The model under review builds one solid part; all positions refer to its coordinate system, in mm. Face numbers are marked on the shaded views. A direction names the side the tool comes from. Coordinates: 2 decimals unless noted, no trailing zeros. Order: outer loops, then holes, each group sorted by start corner. A loop starts at its lowest first (then second) coordinate and runs counter-clockwise, first axis right, second up. Notation, with made-up numbers: M -8,28 L 16,28 A13 ccw 16,52 Z; hole C 28.25,77 d4. An arc over 180 degrees is marked long. One line per item, written item: value.
Autodesk Inventor part; units mm, degrees
ref_plane "YZ Plane" through (0, 0, 0) normal (1, 0, 0) x (0, 1, 0)
ref_plane "XY Plane" through (0, 0, 0) normal (0, 0, 1) x (1, 0, 0)
sketch "Sketch1" plane through (0, 0, 0) normal (0, 0, 1) x (1, 0, 0)
  circle A0 centre (10.05, 11) radius 1.75
  arc A1 (13.575, 6.828427) -> (12.575, 7) centre (12.575, 4) ccw
  line L0 (13.575, 25.055513) -> (13.575, 6.828427)
  arc A2 (13.582607, 25.229787) -> (13.575, 25.055513) centre (15.575, 25.055513) ccw
  arc A3 (12.575, 25.055513) -> (13.582607, 25.229787) centre (12.575, 28.055513) ccw
  line L1 (7.525, 25.055513) -> (12.575, 25.055513)
  arc A4 (6.525, 25.227086) -> (7.525, 25.055513) centre (7.525, 28.055513) ccw
  line L2 (6.525, 6.828427) -> (6.525, 25.227086)
  arc A5 (7.525, 7) -> (6.525, 6.828427) centre (7.525, 4) ccw
  line L3 (12.575, 7) -> (7.525, 7)
  circle A6 centre (10.05, 21.055513) radius 1.75
  line L4 (10.05, 18.055513) -> (22.075, 18.055513)
  line L5 (22.075, 18.055513) -> (22.075, 56.065748)
  circle A7 centre (18.075, 30.055513) radius 1.75
  circle A8 centre (59, 30.055513) radius 1.75
  circle A9 centre (50.975, 2) radius 1.75
  circle A10 centre (10.05, 2) radius 1.75
  line L6 (3.525, -2) -> (3.525, 34.055513)
  arc A11 (3.525, -2) -> (63.525, -2) centre (33.525, 16.027756) ccw
  line L7 (63.525, 34.055513) -> (63.525, -2)
  arc A12 (63.525, 34.055513) -> (3.525, 34.055513) centre (33.525, 16.027756) ccw
  arc A13 (30.525, 56.680798) -> (-6.475, 36.055513) centre (29.281483, 15.411497) ccw
  arc A14 (30.525, 58.681663) -> (-8.207051, 37.055513) centre (29.281483, 15.411497) ccw
  line L8 (16.075, 54.530422) -> (16.075, 24.055513)
  line L9 (16.075, 24.055513) -> (10.05, 24.055513)
  arc A15 (10.05, 24.055513) -> (10.05, 18.055513) centre (10.05, 21.055513) ccw
  line L10 (-6.475, 36.055513) -> (-8.207051, 37.055513)
  line L11 (30.525, 56.680798) -> (30.525, 58.681663)
  line L12 (15.575, 28.055513) -> (15.575, 32.055513)
  point P0 (0, 0)
  point P1 (30.525, 57.681231)
  dimension "d0" = 6
  dimension "d1" = 6
  dimension "d2" = 3
  dimension "d3" = 2
  dimension "d4" = 2
  dimension "d5" = 0.5
  dimension "d6" = 60
  dimension "d22" = 10
  dimension "d23" = 2
sketch "Sketch1 outline for Extrusion1" plane through (0, 0, 0) normal (0, 0, 1) x (1, 0, 0)
  arc A0 (-6.475, 36.055513) -> (16.075, 54.530422) centre (29.281483, 15.411497) cw
  line L0 (16.075, 54.530422) -> (16.075, 24.055513)
  line L1 (16.075, 24.055513) -> (10.05, 24.055513)
  arc A1 (10.05, 24.055513) -> (10.05, 18.055513) centre (10.05, 21.055513) ccw
  line L2 (10.05, 18.055513) -> (22.075, 18.055513)
  line L3 (22.075, 18.055513) -> (22.075, 56.065748)
  arc A2 (22.075, 56.065748) -> (30.525, 56.680798) centre (29.281483, 15.411497) cw
  line L4 (30.525, 56.680798) -> (30.525, 58.681663)
  arc A3 (30.525, 58.681663) -> (-8.207051, 37.055513) centre (29.281483, 15.411497) ccw
  line L5 (-8.207051, 37.055513) -> (-6.475, 36.055513)
  circle A4 centre (10.05, 21.055513) radius 1.75
extrude "Extrusion1" add sketch "Sketch1 outline for Extrusion1" along normal blind 6
sketch "Sketch2" plane through (0, 0, 0) normal (0, 0, -1) x (-1, 0, 0)
  circle A0 centre (-10.05, 21.055513) radius 1.75
  arc A1 (6.475, 36.055513) -> (-16.075, 54.530422) centre (-29.281483, 15.411497) ccw
  line L0 (8.207051, 37.055513) -> (6.475, 36.055513)
  arc A2 (8.207051, 37.055513) -> (-30.525, 58.681663) centre (-29.281483, 15.411497) ccw
  line L1 (-30.525, 56.680798) -> (-30.525, 58.681663)
  arc A3 (-22.075, 56.065748) -> (-30.525, 56.680798) centre (-29.281483, 15.411497) ccw
  line L2 (-22.075, 18.055513) -> (-22.075, 56.065748)
  line L3 (-10.05, 18.055513) -> (-22.075, 18.055513)
  arc A4 (-10.05, 18.055513) -> (-10.05, 24.055513) centre (-10.05, 21.055513) ccw
  line L4 (-16.075, 24.055513) -> (-10.05, 24.055513)
  line L5 (-16.075, 54.530422) -> (-16.075, 24.055513)
  line L6 (-16.075, 54.530422) -> (-16.075, 24.055513)
  line L7 (-10.05, 18.055513) -> (-22.075, 18.055513)
  line L8 (-19.575, 34.055513) -> (-12.575, 34.055513)
  line L9 (-22.075, 18.055513) -> (-22.075, 56.065748)
  line L10 (-16.075, 37.055513) -> (-22.075, 37.055513)
  line L11 (-22.075, 18.055513) -> (-22.075, 56.065748)
  line L12 (-16.075, 37.055513) -> (-16.075, 54.530422)
  line L13 (-22.075, 37.055513) -> (-22.075, 56.065748)
  point P0 (0, 0)
  point P1 (-16.0625, 18.055513)
  dimension "d20" = 3
extrude "Extrusion2" add sketch "Sketch2" along normal blind 3 contours A1 L5 L10 L2 A3 L1 A2 L0
sketch "Sketch3" plane through (0, 0, 6) normal (0, 0, 1) x (1, 0, 0)
  line L0 (10.05, 18.055513) -> (22.075, 18.055513)
  line L1 (22.075, 18.055513) -> (22.075, 56.065748)
  arc A0 (30.525, 56.680798) -> (22.075, 56.065748) centre (29.281483, 15.411497) ccw
  line L2 (30.525, 56.680798) -> (30.525, 58.681663)
  arc A1 (30.525, 58.681663) -> (-8.207051, 37.055513) centre (29.281483, 15.411497) ccw
  line L3 (-8.207051, 37.055513) -> (-6.475, 36.055513)
  arc A2 (16.075, 54.530422) -> (-6.475, 36.055513) centre (29.281483, 15.411497) ccw
  line L4 (16.075, 54.530422) -> (16.075, 24.055513)
  line L5 (16.075, 24.055513) -> (10.05, 24.055513)
  arc A3 (10.05, 24.055513) -> (10.05, 18.055513) centre (10.05, 21.055513) ccw
  circle A4 centre (10.05, 21.055513) radius 1.75
  line L6 (5.525, 34.055513) -> (19.575, 34.055513)
  line L7 (16.075, 54.530422) -> (16.075, 24.055513)
  line L8 (22.075, 56.065748) -> (22.075, 18.055513)
  line L9 (16.075, 24.055513) -> (16.075, 54.530422)
  line L10 (16.075, 39.055513) -> (22.075, 39.055513)
  point P0 (0, 0)
  point P1 (22.075, 24.055513)
  point P2 (22.075, 34.055513)
  dimension "d19" = 5
extrude "Extrusion3" cut sketch "Sketch3" against normal blind 3 contours L10 L4 A2 L3 A1 L2 A0 L1
sketch "Sketch4" plane through (0, 0, -3) normal (0, 0, -1) x (-1, 0, 0)
  arc A0 (6.475, 36.055513) -> (-16.075, 54.530422) centre (-29.281483, 15.411497) ccw
  line L0 (6.475, 36.055513) -> (8.207051, 37.055513)
  arc A1 (8.207051, 37.055513) -> (-30.525, 58.681663) centre (-29.281483, 15.411497) ccw
  line L1 (-30.525, 58.681663) -> (-30.525, 56.680798)
  arc A2 (-22.075, 56.065748) -> (-30.525, 56.680798) centre (-29.281483, 15.411497) ccw
  arc A3 (-16.075, 54.530422) -> (-22.075, 56.065748) centre (-29.281486, 15.411487) ccw
  arc A4 (-22.075, 56.065748) -> (-30.525, 56.680798) centre (-29.281483, 15.411497) ccw
  line L2 (-22.075, 56.065748) -> (-22.075, 37.055513)
  line L3 (-22.075, 37.055513) -> (-16.075, 37.055513)
  line L4 (-16.075, 37.055513) -> (-16.075, 54.530422)
  point P0 (0, 0)
extrude "Extrusion4" add sketch "Sketch4" along normal blind 20 contours A0 A3 A2 L1 A1 L0
fillet "Fillet1" radius 3 7 edges at (16.075, 54.5304, 0) (22.075, 56.0657, 0) (22.075, 18.0555, 3) (-7.341, 36.5555, 3) (-7.341, 36.5555, -23) (30.525, 57.6812, -23) (30.525, 57.6812, 3)
fillet "Fillet2" radius 3 4 edges at (19.075, 39.0555, 3) (19.075, 39.0555, 6) (19.075, 37.0555, -3) (19.075, 37.0555, 0)
ref_plane "Work Plane1" through (29.281483, 58.699528, 0) normal (0, 1, 0) x (-1, 0, 0)
sketch "Sketch6" plane through (0, 0, -3) normal (0, 0, -1) x (-1, 0, 0)
  line L0 (-16.075, 39.251665) -> (-22.075, 39.251665)
  line L1 (-16.075, 39.251665) -> (-16.075, 50.100446)
  arc A0 (-11.805166, 52.818446) -> (-16.075, 50.100446) centre (-13.075, 50.100446) ccw
  arc A1 (-16.075, 54.530422) -> (-22.075, 56.065748) centre (-29.281486, 15.411487) ccw
  arc A2 (-22.075, 53.467756) -> (-24.745407, 56.449595) centre (-25.075, 53.467756) ccw
  line L2 (-22.075, 53.467756) -> (-22.075, 39.251665)
  arc A3 (-3.525, 34.055513) -> (-63.525, 34.055513) centre (-33.525, 16.027756) ccw
  arc A4 (-16.075, 48.654394) -> (-22.075, 51.211524) centre (-33.525, 16.027756) ccw
  line L3 (-22.075, 53.467756) -> (-22.075, 42.055513)
  arc A5 (-16.075, 50.906081) -> (-22.075, 53.309085) centre (-33.525, 16.027756) ccw
  line L4 (-22.075, 51.211524) -> (-22.075, 53.309085)
  line L5 (-16.075, 50.906081) -> (-16.075, 48.654394)
  line L6 (-16.075, 39.251665) -> (-16.075, 50.100446)
  line L7 (-16.075, 42.055513) -> (-16.075, 50.100446)
  line L8 (-16.075, 50.100446) -> (-22.075, 53.309085)
  arc A6 (-11.805166, 52.818446) -> (-16.075, 54.530422) centre (-29.281483, 15.411497) ccw
  arc A7 (-22.075, 56.065748) -> (-24.745407, 56.449595) centre (-29.281483, 15.411497) ccw
  point P0 (0, 0)
  dimension "d37" = 2
  dimension "d38" = 2
sketch "Sketch6 outline for Extrusion7" plane through (0, 0, -3) normal (0, 0, -1) x (-1, 0, 0)
  arc A0 (-16.075, 50.906081) -> (-22.075, 53.309085) centre (-33.525, 16.027756) ccw
  line L0 (-22.075, 53.309085) -> (-22.075, 39.251665)
  line L1 (-22.075, 39.251665) -> (-16.075, 39.251665)
  line L2 (-16.075, 39.251665) -> (-16.075, 50.906081)
extrude "Extrusion7" add sketch "Sketch6 outline for Extrusion7" along normal blind 8
fillet "Fillet6" radius 1 2 edges at (16.075, 45.0789, -11) (22.075, 46.2804, -11)
equation "\"d1\" = d0"
properties part number "obstacle bumper"
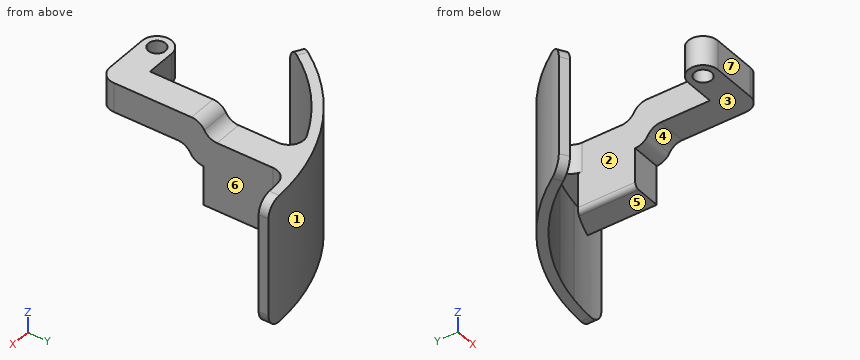
(1) Mouldability with a two-part tool opening along Y and no side actions: class the marked faces 1, 2, 3 and 4 as +Y half, -Y half, draft (parallel to the pull), parting line (faces both ways), or undercut.
Geometry results:
face 1: +Y half
face 2: undercut
face 3: draft
face 4: -Y half
(2) We need section A-A, the plane z = -8.25. State the section outline as (x, y) points (1 decimal).
Geometry results:
outline: M -8.2,37.1 L -6.5,36.1 A41.3 cw 16.1,54.5 A41.3 cw 22.1,56.1 A41.3 cw 30.5,56.7 L 30.5,58.7 A43.3 ccw Z; M 16.1,39.3 L 22.1,39.3 L 22.1,53.3 A39 ccw 16.1,50.9 Z
(3) We need section B-B, the plane x = 11. State the section outline as (y, z) points, plus the area to 3 significant figures.
Geometry results:
outline: M 18.06,0 L 19.59,0 L 19.59,6 L 18.06,6 Z; M 22.53,0 L 24.06,0 L 24.06,6 L 22.53,6 Z; M 52.43,-23 L 54.65,-23 L 54.65,3 L 52.43,3 Z
area: 76.0 mm2
(4) We need section C-C, the plane z = -19. State the section outline as (x, y) points (1 decimal), plus the area to 3 significant figures.
Geometry results:
outline: M -8.2,37.1 L -6.5,36.1 A41.3 cw 16.1,54.5 A41.3 cw 22.1,56.1 A41.3 cw 30.5,56.7 L 30.5,58.7 A43.3 ccw Z
area: 91.1 mm2
(5) For L1, parallel to Y at x = 10.05, z = 1.75; L2, parallel to Z at x = 21.5, y = 24; L3, parallel to Z at x = 2, y = 46.5, list the stretches that pass through material, from the lowest coordinate up.
Geometry results:
L1: y = 18.06 to 19.31, 22.81 to 24.06, 51.95 to 54.19
L2: z = 0 to 6
L3: z = -23 to 3
(6) We need section D-D, the plane y = 29. State the section outline as (x, z) points (3 decimals).
Geometry results:
outline: M 16.075,0 L 22.075,0 L 22.075,6 L 16.075,6 Z
(7) Tool access review of the marked faces 5, 6 and 7: name each direction out of +Z, -Z, +X, -X, +Y, -Y from which nothing blocks a thin tool from reaching the whole face with its end or side.
Geometry results:
face 5: -Z, +X, -Y
face 6: +Z, -Z, +X, -Y
face 7: +Z, -Z, +X, -X, -Y
(8) Insertion check: pin 1 Ø1.9 at (x, y) = (21, 52.5) entering from -Z; pin 2 Ø8 at (x, y) = (20.5, 25) entering from -Z; pin 3 Ø3 at (x, z) = (3.5, -13.5) entering from -Y; pin 4 Ø5 at (y, z) = (35, -3.5) entering from -X. Each pin has a flat end and moves straight along its axis. Give the tip position at first contact, or say it passes through.
Geometry results:
pin 1: stops at z = -11
pin 2: stops at z = 0
pin 3: stops at y = 46.4
pin 4: stops at x = -8.21
